```python
from build123d import *

# Parameters (mm, degrees)
F0_R     = 4
F1_DEPTH = 25.4
F2_R     = 4
F3_DEPTH = 6.35
F4_R     = 4
F5_DEPTH = 6.35
F6_R     = 4
F7_DEPTH = 6.35
F8_R     = 4
F9_DEPTH = 6.35


with BuildPart() as f1:
    # F0 (on Right) → F1 (new body)
    with BuildSketch(Plane.YZ):
        with BuildLine():
            ThreePointArc((203.2, 22.225), (202.270064, 24.470064), (200.025, 25.4))
            Line((200.025, 25.4), (-200.025, 25.4))
            ThreePointArc((-200.025, 25.4), (-202.270064, 24.470064), (-203.2, 22.225))
            Line((-203.2, 22.225), (-203.2, -22.225))
            ThreePointArc((-203.2, -22.225), (-202.270064, -24.470064), (-200.025, -25.4))
            Line((-200.025, -25.4), (200.025, -25.4))
            ThreePointArc((200.025, -25.4), (202.270064, -24.470064), (203.2, -22.225))
            Line((203.2, -22.225), (203.2, 22.225))
        make_face()
        with Locations((-139.7, 0)):
            Circle(F0_R, mode=Mode.SUBTRACT)
        Circle(F0_R, mode=Mode.SUBTRACT)
        with Locations((139.7, 0)):
            Circle(F0_R, mode=Mode.SUBTRACT)
    extrude(amount=F1_DEPTH)

    # F2 (on face) → F3 (cut)
    with BuildSketch(Plane.XZ.offset(203.2)):
        with Locations((12.734205, 0)):
            Circle(F2_R)
    extrude(amount=-F3_DEPTH, mode=Mode.SUBTRACT)

    # F4 (on face) → F5 (cut)
    with BuildSketch(Plane(origin=(0, 203.2, 0), x_dir=(-1, 0, 0), z_dir=(0, 1, 0))):
        with Locations((-12.224027, 0)):
            Circle(F4_R)
    extrude(amount=-F5_DEPTH, mode=Mode.SUBTRACT)

    # F6 (on face) → F7 (cut)
    with BuildSketch(Plane.XY.offset(25.4)):
        with Locations((12.7, -188.595)):
            Circle(F6_R)
    extrude(amount=-F7_DEPTH, mode=Mode.SUBTRACT)

    # F8 (on face) → F9 (cut)
    with BuildSketch(Plane.XY.offset(25.4)):
        with Locations((12.7, 188.595)):
            Circle(F8_R)
    extrude(amount=-F9_DEPTH, mode=Mode.SUBTRACT)


solid = f1.part
```
Could you check a few things on this model? Use its own coordinates, in mm. A direction names the side the tool comes from. Coordinates: 2 decimals unless noted, no trailing zeros. Write each loop counter-clockwise with the first axis right and the second up, starting at its lowest first coordinate (ties: lowest second). Pieces come first, ordered by that corner, then holes. Notation, with made-up numbers: (82.25, 78.5) -> (124.25, 78.5) arc R37 ccw to (124.25, 117.5) -> close; hole circle Ø11 at (-12, 50.5). An arc over 180 degrees is marked (long way). Return JSON: item names as keys, results as strings.
(1) Imagine slicing it at A-A, the plane y = 139.7. Please give me the cut outline in (x, z).
Numbers:
{"outline": "(0, -25.4) -> (25.4, -25.4) -> (25.4, -4) -> (0, -4) -> close; (0, 4) -> (25.4, 4) -> (25.4, 25.4) -> (0, 25.4) -> close"}
(2) We'd pull the mould along Z, two halves only. Please class faces 6 (the flat face through (13, -203.2, 5)), 7 (the flat face through (13, 3, 25.4)), 8 (the cylindrical face through (12.52, 136.75, 2.7)): +Z half, -Z half, draft (parallel to the pull), parting line (faces both ways), or undercut.
Numbers:
{"face 6": "draft", "face 7": "+Z half", "face 8": "undercut"}
(3) Imagine slicing it at B-B, the plane x = 12.7. Please give me the cut outline in (y, z) (3 decimals).
Numbers:
{"outline": "(-203.2, -22.225) arc R3.175 ccw to (-200.025, -25.4) -> (200.025, -25.4) arc R3.175 ccw to (203.2, -22.225) -> (203.2, -3.972) -> (196.85, -3.972) -> (196.85, 3.972) -> (203.2, 3.972) -> (203.2, 22.225) arc R3.175 ccw to (200.025, 25.4) -> (192.595, 25.4) -> (192.595, 19.05) -> (184.595, 19.05) -> (184.595, 25.4) -> (-184.595, 25.4) -> (-184.595, 19.05) -> (-192.595, 19.05) -> (-192.595, 25.4) -> (-200.025, 25.4) arc R3.175 ccw to (-203.2, 22.225) -> (-203.2, 4) -> (-196.85, 4) -> (-196.85, -4) -> (-203.2, -4) -> close; hole circle Ø8 at (-139.7, 0); hole circle Ø8 at (0, 0); hole circle Ø8 at (139.7, 0)"}
(4) I'm going to push flat-ended pins straight in: pin 1 (4 mm diameter, centred on x = 14.5, y = 189, fed in from +Z); pin 2 (4 mm diameter, centred on x = 12.5, z = 0, fed in from -Y); pin 3 (6.5 mm diameter, centred on x = 12.22, z = 0, fed in from +Y). Where does each tip first touch, or does it pass through?
Numbers:
{"pin 1": "stops at z = 19.05", "pin 2": "stops at y = -196.85", "pin 3": "stops at y = 196.85"}
(5) Which directions (+Z, -Z, +X, -X, +Y, -Y) give clear straight access to the entire face, cutting with the end or side of a thin tool? Please do faces 1 (the cylindrical face through (11.867, -200.069, -3.905)), 2 (the cylindrical face through (12.522, -0.867, -3.905)), 3 (the flat face through (0, -3, 6)), 4 (the cylindrical face through (11.83, 184.69, 22.27)), 5 (the flat face through (12, 196.85, 0)).
Numbers:
{"face 1": "-Y", "face 2": "+X, -X", "face 3": "+Z, -Z, -X, +Y, -Y", "face 4": "+Z", "face 5": "+Y"}
(6) I need wall thicknesses on L1, parallel to Y at x = 12.7, z = 21 (3 decimals); L2, parallel to Y at x = 17.25, z = -0.5; L3, parallel to Y at x = 12.7, z = 24 (3 decimals). Which ranges of each line are inside material? Lowest first, please.
Numbers:
{"L1": "y = -203.2 to -192.595, -184.595 to 184.595, 192.595 to 203.2", "L2": "y = -203.2 to -143.67, -135.73 to -3.97, 3.97 to 135.73, 143.67 to 203.2", "L3": "y = -202.657 to -192.595, -184.595 to 184.595, 192.595 to 202.657"}
